Could you check a few things on this drawing? It's one solid part, dimensions in mm from its lowest x, y, z. Coordinates: 2 decimals unless noted, no trailing zeros. Order: outer loops, then holes, each group sorted by start corner. A loop starts at its lowest first (then second) coordinate and runs counter-clockwise, first axis right, second up. Notation, with made-up numbers: (31.5, 34.5) -> (89.5, 34.5) arc R29 cw to (89.5, 63.5) -> close; hole circle Ø8 at (-9, 81.25). An arc over 180 degrees is marked (long way). Use a Markdown table: item, result. Add a question column.
1. If I drill on line 1 along Y through (x, z) = (88.7, 1.15) (1 decimal); line 2 along X through (y, z) = (64.7, 1.9) (1 decimal); line 3 along Y through (x, z) = (12.7, 1.9) (1 decimal), over which ranges is the centre line in solid material (lowest first)? Write a range as from..to.
2. Suppose I cut it at A-A, the plane x = 88.7. List the corners of the cut face in (y, z) for me (1 decimal).
3. Suppose I cut it at B-B, the plane y = 12.7. List the corners of the cut face in (x, z) for me (1 decimal), then the cut area to 3 significant figures.
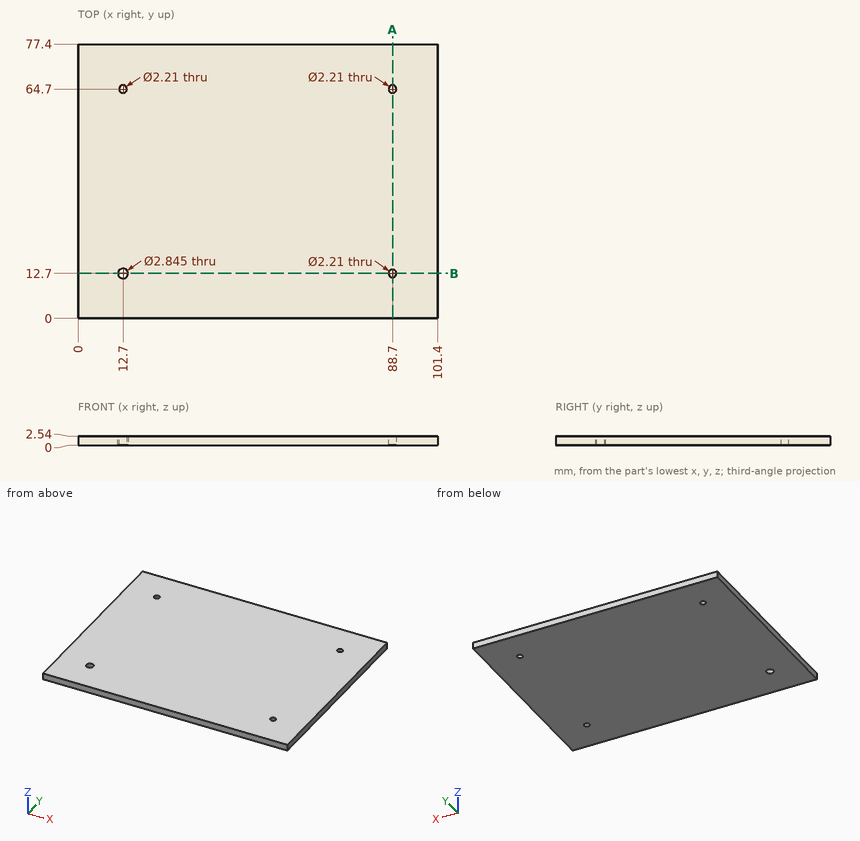
Worked out:
| question | item | result |
|---|---|---|
| 1 | line 1 | y = 0..11.6, 13.8..63.6, 65.8..77.4 |
| 1 | line 2 | x = 0..11.6, 13.8..87.6, 89.8..101.4 |
| 1 | line 3 | y = 0..11.3, 14.1..63.6, 65.8..77.4 |
| 2 | outline | (0, 0) -> (11.6, 0) -> (11.6, 2.5) -> (0, 2.5) -> close; (13.8, 0) -> (63.6, 0) -> (63.6, 2.5) -> (13.8, 2.5) -> close; (65.8, 0) -> (77.4, 0) -> (77.4, 2.5) -> (65.8, 2.5) -> close |
| 3 | outline | (0, 0) -> (11.3, 0) -> (11.3, 2.5) -> (0, 2.5) -> close; (14.1, 0) -> (87.6, 0) -> (87.6, 2.5) -> (14.1, 2.5) -> close; (89.8, 0) -> (101.4, 0) -> (101.4, 2.5) -> (89.8, 2.5) -> close |
| 3 | area | 245 mm² |
